The model under review builds one solid part; all positions refer to its coordinate system, in mm. A direction names the side the tool comes from. Coordinates: 2 decimals unless noted, no trailing zeros. Order: outer loops, then holes, each group sorted by start corner. A loop starts at its lowest first (then second) coordinate and runs counter-clockwise, first axis right, second up. Notation, with made-up numbers: (62, 86) -> (73, 86) arc R11 cw to (73, 97) -> close; hole circle Ø6 at (-11.75, 79.25). An arc over 180 degrees is marked (long way). Put each result on its own line as item: value.
from build123d import *

# Parameters (mm, degrees)
SKETCH2_W           = 79.4
SKETCH2_H           = 121.8
BOSS_EXTRUDE1_DEPTH = 10
CUT_EXTRUDE1_DEPTH  = 3
SKETCH7_W           = 66.4
SKETCH7_H           = 111.011877984
CUT_EXTRUDE4_DEPTH  = 7.5
FILLET2_R           = 2
SKETCH6_R           = 1.75
CUT_EXTRUDE5_DEPTH  = 26.5


with BuildPart() as part:
    # Sketch2 → Boss-Extrude1 (new body)
    with BuildSketch(Plane(origin=(0, 0, 0), x_dir=(0, 0, -1), z_dir=(1, 0, 0))):
        with Locations((0, 39.742697631)):
            Rectangle(SKETCH2_W, SKETCH2_H)
    extrude(amount=BOSS_EXTRUDE1_DEPTH)

    # Sketch3 → Cut-Extrude1 (cut)
    with BuildSketch(Plane(origin=(0, 0, 0), x_dir=(0, 0, -1), z_dir=(1, 0, 0))):
        with BuildLine():
            Line((-38.7, 1.942697631), (-38.7, 2.940614447))
            Line((-38.7, 2.940614447), (-37.3, 2.940614447))
            Line((-37.3, 2.940614447), (-37.3, 98.342697631))
            ThreePointArc((-37.3, 98.342697631), (-36.919238816, 99.261936446), (-36, 99.642697631))
            Line((-36, 99.642697631), (36, 99.642697631))
            ThreePointArc((36, 99.642697631), (36.919238816, 99.261936446), (37.3, 98.342697631))
            Line((37.3, 98.342697631), (37.3, 2.940614447))
            Line((37.3, 2.940614447), (38.7, 2.940614447))
            Line((38.7, 2.940614447), (38.7, 1.942697631))
            Line((38.7, 1.942697631), (38.7, -20.157302369))
            Line((38.7, -20.157302369), (-38.7, -20.157302369))
            Line((-38.7, -20.157302369), (-38.7, 1.942697631))
        make_face()
        Polygon((-34.7, -15.857302369), (-34.7, -16.969180353), (34.7, -16.969180353), (34.7, -15.857302369), (34.7, -1.057302369), (34.7, -0.657302369), (34.7, 97.042697631), (-34.7, 97.042697631), (-34.7, -0.657302369), (-34.7, -1.057302369), align=None, mode=Mode.SUBTRACT)
    extrude(amount=CUT_EXTRUDE1_DEPTH, mode=Mode.SUBTRACT)

    # Sketch7 → Cut-Extrude4 (cut)
    with BuildSketch(Plane.ZY):
        with Locations((0, 40.036758639)):
            Rectangle(SKETCH7_W, SKETCH7_H)
    extrude(amount=-CUT_EXTRUDE4_DEPTH, mode=Mode.SUBTRACT)

    # Fillet2
    fillet2_edges = [part.edges().sort_by_distance(p)[0] for p in [
        (10, 39.742697631, -39.7),
        (10, 100.642697631, 0),
        (1.5, -16.969180353, 34.7),
        (1.5, -16.969180353, -34.7),
        (10, 39.742697631, 39.7),
        (7.5, -15.469180353, 0),
        (3.75, -15.469180353, 33.2),
        (7.5, 40.036758639, 33.2),
        (3.75, 95.542697631, 33.2),
        (7.5, 95.542697631, 0),
        (3.75, 95.542697631, -33.2),
        (7.5, 40.036758639, -33.2),
        (3.75, -15.469180353, -33.2),
        (10, -21.157302369, 0),
        (5, 100.642697631, 39.7),
        (5, 100.642697631, -39.7),
    ]]
    fillet(fillet2_edges, radius=FILLET2_R)

    # Sketch6 → Cut-Extrude5 (cut)
    with BuildSketch(Plane(origin=(10, 0, 0), x_dir=(0, 0, -1), z_dir=(1, 0, 0))):
        with Locations((-28.7, 91)):
            Circle(SKETCH6_R)
        with Locations((25.2, 91)):
            Circle(SKETCH6_R)
        with Locations((-28.7, 71)):
            Circle(SKETCH6_R)
        with Locations((-28.7, 51)):
            Circle(SKETCH6_R)
        with Locations((-28.7, 31)):
            Circle(SKETCH6_R)
        with Locations((25.2, 31)):
            Circle(SKETCH6_R)
        with Locations((25.2, 51)):
            Circle(SKETCH6_R)
        with Locations((25.2, 71)):
            Circle(SKETCH6_R)
        with Locations((-28.7, 15)):
            Circle(SKETCH6_R)
        with Locations((25.2, 15)):
            Circle(SKETCH6_R)
        with Locations((-28.7, -5)):
            Circle(SKETCH6_R)
        with Locations((25.2, -5)):
            Circle(SKETCH6_R)
    extrude(amount=-CUT_EXTRUDE5_DEPTH, mode=Mode.SUBTRACT)


solid = part.part
Item 1: Consider section C-C on z = 13. Write out the cut boundary in (x, y).
Answers below:
outline: (0, -21.16) -> (8, -21.16) arc R2 ccw to (10, -19.16) -> (10, 98.64) arc R2 ccw to (8, 100.64) -> (0, 100.64) -> (0, 99.64) -> (3, 99.64) -> (3, 97.04) -> (0, 97.04) -> (0, 95.54) -> (5.5, 95.54) arc R2 cw to (7.5, 93.54) -> (7.5, -13.47) arc R2 cw to (5.5, -15.47) -> (0, -15.47) -> (0, -16.97) -> (3, -16.97) -> (3, -20.16) -> (0, -20.16) -> close
Item 2: Mouldability with a two-part tool opening along Y and no side actions: class faces 3 (the flat face through (4, -21.157, 1)), 4 (the flat face through (4, 38, -39.7)), 5 (the flat face through (1, 42, -34.7)) as +Y half, -Y half, draft (parallel to the pull), parting line (faces both ways), or undercut.
Answers below:
face 3: -Y half
face 4: draft
face 5: undercut
Item 3: Consider section B-B on y = 91. Write out the cut boundary in (x, z), and give its area (3 significant figures).
Answers below:
outline: (0, -39.7) -> (8, -39.7) arc R2 ccw to (10, -37.7) -> (10, -26.95) -> (7.5, -26.95) -> (7.5, -31.2) arc R2 cw to (5.5, -33.2) -> (0, -33.2) -> (0, -34.7) -> (3, -34.7) -> (3, -37.3) -> (0, -37.3) -> close; (0, 33.2) -> (5.5, 33.2) arc R2 cw to (7.5, 31.2) -> (7.5, 30.45) -> (10, 30.45) -> (10, 37.7) arc R2 ccw to (8, 39.7) -> (0, 39.7) -> (0, 37.3) -> (3, 37.3) -> (3, 34.7) -> (0, 34.7) -> close; (7.5, -23.45) -> (10, -23.45) -> (10, 26.95) -> (7.5, 26.95) -> close
area: 263 mm^2
Item 4: Consider section D-D on y = 36.5. Write out the cut boundary in (x, z), and give its area (3 significant figures).
Answers below:
outline: (0, -39.7) -> (8, -39.7) arc R2 ccw to (10, -37.7) -> (10, 37.7) arc R2 ccw to (8, 39.7) -> (0, 39.7) -> (0, 37.3) -> (3, 37.3) -> (3, 34.7) -> (0, 34.7) -> (0, 33.2) -> (5.5, 33.2) arc R2 cw to (7.5, 31.2) -> (7.5, -31.2) arc R2 cw to (5.5, -33.2) -> (0, -33.2) -> (0, -34.7) -> (3, -34.7) -> (3, -37.3) -> (0, -37.3) -> close
area: 280 mm^2
Item 5: For pin 1 Ø5.5 at (y, z) = (91, -25.2) entering from -X; pin 2 Ø4.5 at (y, z) = (71, 28.7) entering from +X, all flat-tipped, find the tip position at first contact; note any pin that passes through.
Answers below:
pin 1: x = 7.49
pin 2: x = 10
Item 6: For faces 1 (the flat face through (1, -16.969, 0)), 2 (the cylindrical face through (8.768, 90.33, 27.083)), list the 3-axis set-ups (+Z, -Z, +X, -X, +Y, -Y) from which the entire face can be reached by the end or side of a thin tool; tool diameter is ignored.
Answers below:
face 1: -X
face 2: +X, -X
Item 7: Consider section A-A on y = -5. Write out the cut boundary in (x, z).
Answers below:
outline: (0, -39.7) -> (8, -39.7) arc R2 ccw to (10, -37.7) -> (10, -26.95) -> (7.5, -26.95) -> (7.5, -31.2) arc R2 cw to (5.5, -33.2) -> (0, -33.2) -> (0, -34.7) -> (3, -34.7) -> (3, -38.7) -> (0, -38.7) -> close; (0, 33.2) -> (5.5, 33.2) arc R2 cw to (7.5, 31.2) -> (7.5, 30.45) -> (10, 30.45) -> (10, 37.7) arc R2 ccw to (8, 39.7) -> (0, 39.7) -> (0, 38.7) -> (3, 38.7) -> (3, 34.7) -> (0, 34.7) -> close; (7.5, -23.45) -> (10, -23.45) -> (10, 26.95) -> (7.5, 26.95) -> close
Item 8: For line 1 (Y direction, x = 1.75, z = -28); line 2 (Z direction, x = 8.65, y = 91); line 3 (Y direction, x = 4.75, z = -25), list the stretches that pass through material, from the lowest coordinate up. Write a range as from..to.
Answers below:
line 1: -21.16..-20.16, -16.97..-15.47, 95.54..97.04, 99.64..100.64
line 2: -39.59..-26.95, -23.45..26.95, 30.45..39.59
line 3: -21.16..-15.47, 95.54..100.64
